The listing builds one solid part. Answer for the finished solid, in the listing's coordinates (mm). A direction names the side the tool comes from. Coordinates: 2 decimals unless noted, no trailing zeros. Loops run counter-clockwise (first coordinate to the right, second up) from the corner with the lowest first, then second, coordinate; pieces in that order, holes last. Notation, with made-up numbers: (18, 62) - (69, 62) arc R26 cw to (69, 88) - close; hole circle Ø8 at (89, 63). An arc over 180 degrees is marked (long way). Return JSON: item names as keys, results as strings. Group by question number.
1. The mould has two halves that part along Z. Classify faces 1 (the face through (-1, 3, -45)), 2 (the face through (-36, 3, 1)), 3 (the face through (27.4, 2.6, 36.4)): pulls with the +Z half, pulls with the -Z half, needs draft (parallel to the pull), parting line crosses it, or undercut.
2. Which of the six approach directions +Z, -Z, +X, -X, +Y, -Y give full straight-line access (tool end or side, diameter ignored) to faces 4 (the face through (-26.74, 1.28, 36.42)), 5 (the face through (25.295, 4.324, 38.173))?
3. Section B-B (x = 26) is taken. Write down the section's boundary in (y, z).
4. Section C-C (z = 19) is taken. Write down the section's boundary in (x, y).
5. This flat-tipped pin is pushed along its axis until it touches: P1, Ø4, axis at x = 26, z = 35, coming from the +Y side. Where does it stop, or does it pass through?
6. Section A-A (z = -35) is taken. Write down the section's boundary in (x, y), and give its area (3 significant figures).
7. Find the intervals of material crossed by line 1 along Z through (x, y) = (-12, 3); line 2 along X through (y, z) = (4.75, 35); line 3 along Z through (x, y) = (26, 5.05), in increasing order.
8. Section D-D (y = 4.45) is taken. Write down the section's boundary in (x, z).
```python
from build123d import *

# Parameters (mm, degrees)
SZKIC1_W                                            = 72
SZKIC1_H                                            = 90
DODANIE_WYCI_GNI_CIE1_DEPTH                         = 6
CBORE_FOR_M3_HEX_SOCKET_HEAD_CAP_SCREW1_D           = 3.2
CBORE_FOR_M3_HEX_SOCKET_HEAD_CAP_SCREW1_DEPTH       = 7.7
CBORE_FOR_M3_HEX_SOCKET_HEAD_CAP_SCREW1_CBORE_D     = 6.5
CBORE_FOR_M3_HEX_SOCKET_HEAD_CAP_SCREW1_CBORE_DEPTH = 3.4
CBORE_FOR_M3_HEX_SOCKET_HEAD_CAP_SCREW1_TIP         = 0.96137699
F_1_0MM_DOWEL_HOLE1_D                               = 3.9


with BuildPart() as part:
    # Szkic1 → Dodanie-wyciągnięcie1 (new body)
    with BuildSketch(Plane(origin=(0, 0, 0), x_dir=(1, 0, 0), z_dir=(0, 1, 0))):
        Rectangle(SZKIC1_W, SZKIC1_H)
    extrude(amount=DODANIE_WYCI_GNI_CIE1_DEPTH)

    # CBORE for M3 Hex Socket Head Cap Screw1
    with Locations(Plane(origin=(0, 6, 0), x_dir=(1, 0, 0), z_dir=(0, 1, 0))):
        with Locations((-26, 35), (26, 35), (26, -35), (-26, -35)):
            CounterBoreHole(CBORE_FOR_M3_HEX_SOCKET_HEAD_CAP_SCREW1_D / 2, CBORE_FOR_M3_HEX_SOCKET_HEAD_CAP_SCREW1_CBORE_D / 2, CBORE_FOR_M3_HEX_SOCKET_HEAD_CAP_SCREW1_CBORE_DEPTH, depth=CBORE_FOR_M3_HEX_SOCKET_HEAD_CAP_SCREW1_DEPTH)
            with Locations((0, 0, -(CBORE_FOR_M3_HEX_SOCKET_HEAD_CAP_SCREW1_DEPTH + CBORE_FOR_M3_HEX_SOCKET_HEAD_CAP_SCREW1_TIP / 2))):  # 118° drill point
                Cone(0, CBORE_FOR_M3_HEX_SOCKET_HEAD_CAP_SCREW1_D / 2, CBORE_FOR_M3_HEX_SOCKET_HEAD_CAP_SCREW1_TIP, mode=Mode.SUBTRACT)

    # Ø1.0mm Dowel Hole1 (through all)
    with Locations(Plane(origin=(0, 6, 0), x_dir=(1, 0, 0), z_dir=(0, 1, 0))):
        with Locations((-12, -19), (-12, 19)):
            Hole(F_1_0MM_DOWEL_HOLE1_D / 2)


solid = part.part
```
The answers:
{
 "1": {"face 1": "pulls with the -Z half", "face 2": "needs draft", "face 3": "undercut"},
 "2": {"face 4": "+Y, -Y", "face 5": "+Y"},
 "3": {"outline": "(0, -45) - (6, -45) - (6, -38.25) - (2.6, -38.25) - (2.6, -36.6) - (0, -36.6) - close; (0, -33.4) - (2.6, -33.4) - (2.6, -31.75) - (6, -31.75) - (6, 31.75) - (2.6, 31.75) - (2.6, 33.4) - (0, 33.4) - close; (0, 36.6) - (2.6, 36.6) - (2.6, 38.25) - (6, 38.25) - (6, 45) - (0, 45) - close"},
 "4": {"outline": "(-36, 0) - (-13.95, 0) - (-13.95, 6) - (-36, 6) - close; (-10.05, 0) - (36, 0) - (36, 6) - (-10.05, 6) - close"},
 "5": {"P1": "stops at y = 2.6"},
 "6": {"outline": "(-36, 0) - (-27.6, 0) - (-27.6, 2.6) - (-29.25, 2.6) - (-29.25, 6) - (-36, 6) - close; (-24.4, 0) - (24.4, 0) - (24.4, 2.6) - (22.75, 2.6) - (22.75, 6) - (-22.75, 6) - (-22.75, 2.6) - (-24.4, 2.6) - close; (27.6, 0) - (36, 0) - (36, 6) - (29.25, 6) - (29.25, 2.6) - (27.6, 2.6) - close", "area": "371 mm2"},
 "7": {"line 1": "z = -45 to -20.95, -17.05 to 17.05, 20.95 to 45", "line 2": "x = -36 to -29.25, -22.75 to 22.75, 29.25 to 36", "line 3": "z = -45 to -38.25, -31.75 to 31.75, 38.25 to 45"},
 "8": {"outline": "(-36, -45) - (36, -45) - (36, 45) - (-36, 45) - close; hole circle Ø6.5 at (-26, -35); hole circle Ø6.5 at (-26, 35); hole circle Ø3.9 at (-12, -19); hole circle Ø3.9 at (-12, 19); hole circle Ø6.5 at (26, -35); hole circle Ø6.5 at (26, 35)"}
}
